Input: part model. Units: mm. Frame: model coordinates. Face numbers are marked on the shaded views. Coordinates: 2 decimals unless noted, no trailing zeros. Loops run counter-clockwise (first coordinate to the right, second up) from the corner with the lowest first, then second, coordinate; pieces in that order, holes last.
(1) Section B-B, the plane z = 4. Return loops of the section in (x, y), then the cut area to 3 significant figures.
(2) Section C-C, the plane y = 1.5. Return loops of the section in (x, z), then the cut area to 3 significant figures.
(3) Contact query for a flat-ended pin moving along its axis: P1, Ø3, axis at x = -7, y = 0, coming from the -Z side. Output: stop coordinate, or through.
(4) Mould query, pull axis X, two halves, no side actions, for the marked faces 1, 2 and 3. Classes: released by +X, released by -X, zero draft, split by the parting line, or undercut.
(5) Section A-A, the plane x = 6. Return loops of the section in (y, z).
(6) Section D-D, the plane x = -7. Return loops of the section in (y, z), then the cut area to 3 significant figures.
(7) Line query: L1, parallel to Y at x = -7, z = 8.75; L2, parallel to Z at x = -5, y = 3.75; L3, parallel to Y at x = -7, z = 1.05. Output: solid intervals per line, ascending.
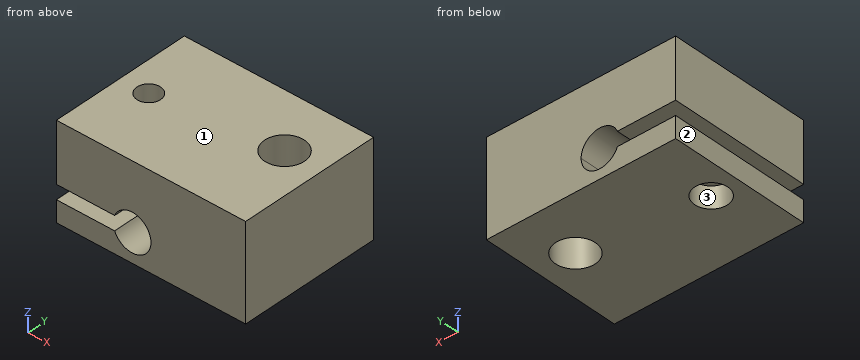
```python
from build123d import *

# Parameters (mm, degrees)
F0_W     = 20
F0_H     = 15
F1_DEPTH = 10
F3_D     = 4.2
F5_DEPTH = 15.001
F7_D     = 3.5
F7_DEPTH = 3
F7_TIP   = 1.0515060833
F9_D     = 2.5


with BuildPart() as f1:
    # F0 (on Top) → F1 (new body)
    with BuildSketch(Plane.XY):
        Rectangle(F0_W, F0_H)
    extrude(amount=F1_DEPTH)

    # F3 (through all)
    with Locations(Plane.XY.offset(10)):
        with Locations((6, 1.5)):
            Hole(F3_D / 2)

    # F4 (on face) → F5 (cut, through all)
    with BuildSketch(Plane.XZ.offset(7.5)):
        with BuildLine():
            ThreePointArc((-3.8446359594, 2.25), (-1.6178994152, 1.0457275099), (-0.0087235695, 3))
            ThreePointArc((-0.0087235695, 3), (-1.6178994152, 4.9542724901), (-3.8446359594, 3.75))
            ThreePointArc((-3.8446359594, 3.75), (-3.9912764305, 3), (-3.8446359594, 2.25))
        make_face()
        with BuildLine():
            ThreePointArc((-3.8446359594, 2.25), (-3.9912764305, 3), (-3.8446359594, 3.75))
            Line((-3.8446359594, 3.75), (-10, 3.75))
            Line((-10, 3.75), (-10, 2.25))
            Line((-10, 2.25), (-3.8446359594, 2.25))
        make_face()
    extrude(amount=-F5_DEPTH, mode=Mode.SUBTRACT)

    # F7
    with Locations(Plane(origin=(0, 0, 0), x_dir=(1, 0, 0), z_dir=(0, 0, -1))):
        with Locations((-7, 0)):
            Hole(F7_D / 2, depth=F7_DEPTH)
            with Locations((0, 0, -(F7_DEPTH + F7_TIP / 2))):  # 118° drill point
                Cone(0, F7_D / 2, F7_TIP, mode=Mode.SUBTRACT)

    # F9 (through all)
    with Locations(Plane.XY.offset(10)):
        with Locations((-7, 0)):
            Hole(F9_D / 2)


solid = f1.part
```
Report:
1. outline: (-10, -7.5) - (-3.72, -7.5) - (-3.72, 7.5) - (-10, 7.5) - close; (-0.28, -7.5) - (10, -7.5) - (10, 7.5) - (-0.28, 7.5) - close; hole circle Ø2.5 at (-7, 0); hole circle Ø4.2 at (6, 1.5)
1. area: 230 mm2
2. outline: (-10, 0) - (-7.9, 0) - (-7.9, 2.25) - (-10, 2.25) - close; (-10, 3.75) - (-3.84, 3.75) arc R1.99 cw (long way) to (-3.84, 2.25) - (-6.1, 2.25) - (-6.1, 0) - (3.9, 0) - (3.9, 10) - (-10, 10) - close; (8.1, 0) - (10, 0) - (10, 10) - (8.1, 10) - close
2. area: 132 mm2
3. P1: stops at z = 3.75
4. face 1: zero draft
4. face 2: released by -X
4. face 3: undercut
5. outline: (-7.5, 0) - (-0.6, 0) - (-0.6, 10) - (-7.5, 10) - close; (3.6, 0) - (7.5, 0) - (7.5, 10) - (3.6, 10) - close
6. outline: (-7.5, 0) - (-1.75, 0) - (-1.75, 2.25) - (-7.5, 2.25) - close; (-7.5, 3.75) - (-1.25, 3.75) - (-1.25, 10) - (-7.5, 10) - close; (1.25, 3.75) - (7.5, 3.75) - (7.5, 10) - (1.25, 10) - close; (1.75, 0) - (7.5, 0) - (7.5, 2.25) - (1.75, 2.25) - close
6. area: 104 mm2
7. L1: y = -7.5 to -1.25, 1.25 to 7.5
7. L2: z = 0 to 2.25, 3.75 to 10
7. L3: y = -7.5 to -1.75, 1.75 to 7.5
